The drawing under review shows one solid part. Ordinate dimensions are in mm from its lowest x, y, z. A direction names the side the tool comes from. Round coordinates to 2 decimals unless told otherwise and drop trailing zeros. Write each loop counter-clockwise with the first axis right and the second up, starting at its lowest first coordinate (ties: lowest second). Pieces come first, ordered by that corner, then holes.
Item 1: Add section D-D (z = 8). Give the boundary of the cut face in (x, y).
Item 2: Machinability: for the marked faces 4, 5, 6 and 7, which of the approach directions +Z, -Z, +X, -X, +Y, -Y give a long, thin tool a straight path to every point of the face, cutting with its end or side? Answer none if there is none.
Item 3: Draft analysis for pull direction Y (two halves, no side actions). For the marked faces 1, 2 and 3, state which applies: +Y half, -Y half, draft (parallel to the pull), parting line (faces both ways), or undercut.
Item 4: Add section C-C (x = 10.5). Give the boundary of the cut face in (y, z).
Item 5: Add section B-B (y = 8). Give the boundary of the cut face in (x, z), plus the area to 3 significant figures.
Item 6: Add section A-A (z = 1). Give the boundary of the cut face in (x, y) (1 decimal).
Item 7: To check wall thickness, follow L1, parallel to Y at x = 8, z = 1.3; L2, parallel to Z at x = 9, y = 14. State the ranges of each line that lie inside material, in increasing order.
Item 8: Clearance check with flat-ended pins moving along their axes: pin 1 Ø3 at (y, z) = (14, 6.5) entering from +X; pin 2 Ø4 at (x, y) = (11.5, 4.5) entering from +Z; pin 3 Ø3 at (y, z) = (1.5, 5.5) entering from -X. State where each tip first meets the part, or that it passes through.
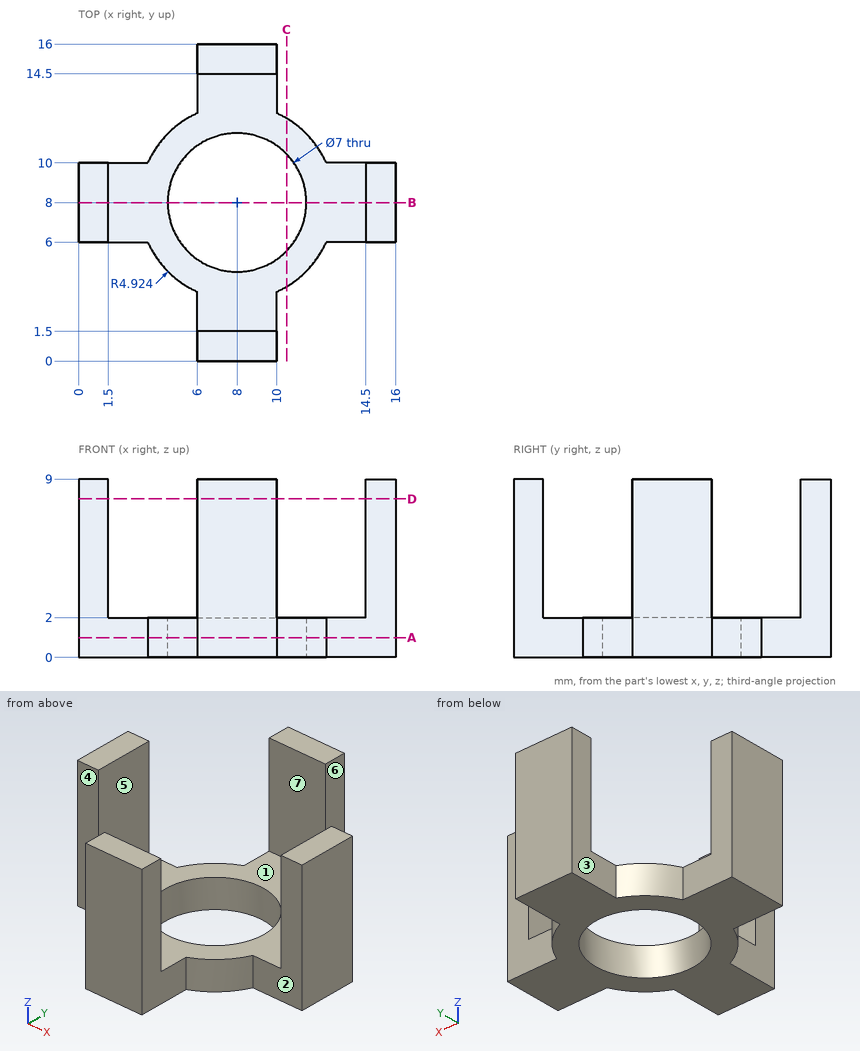
Numbers:
1. outline: (0, 6) - (1.5, 6) - (1.5, 10) - (0, 10) - close; (6, 0) - (10, 0) - (10, 1.5) - (6, 1.5) - close; (6, 14.5) - (10, 14.5) - (10, 16) - (6, 16) - close; (14.5, 6) - (16, 6) - (16, 10) - (14.5, 10) - close
2. face 4: +Z, -Z, -X, -Y
2. face 5: +Z, +Y, -Y
2. face 6: +Z, -Z, +X, +Y
2. face 7: +Z, +X, -X
3. face 1: undercut
3. face 2: -Y half
3. face 3: draft
4. outline: (3.76, 0) - (5.55, 0) - (5.55, 2) - (3.76, 2) - close; (10.45, 0) - (12.24, 0) - (12.24, 2) - (10.45, 2) - close
5. outline: (0, 0) - (4.5, 0) - (4.5, 2) - (1.5, 2) - (1.5, 9) - (0, 9) - close; (11.5, 0) - (16, 0) - (16, 9) - (14.5, 9) - (14.5, 2) - (11.5, 2) - close
5. area: 39.0 mm2
6. outline: (0, 6) - (3.5, 6) arc R4.9 ccw to (6, 3.5) - (6, 0) - (10, 0) - (10, 3.5) arc R4.9 ccw to (12.5, 6) - (16, 6) - (16, 10) - (12.5, 10) arc R4.9 ccw to (10, 12.5) - (10, 16) - (6, 16) - (6, 12.5) arc R4.9 ccw to (3.5, 10) - (0, 10) - close; hole circle Ø7 at (8, 8)
7. L1: y = 0 to 4.5, 11.5 to 16
7. L2: z = 0 to 2
8. pin 1: stops at x = 10
8. pin 2: stops at z = 2
8. pin 3: stops at x = 6
